Source: CAD feature listing. Evaluate the final solid. Frame: model axes, mm. Face numbers are marked on the shaded views. A direction names the side the tool comes from. Coordinates: 2 decimals unless noted, no trailing zeros. Loops run counter-clockwise (first coordinate to the right, second up) from the corner with the lowest first, then second, coordinate; pieces in that order, holes last. Notation, with made-up numbers: (59.5, -11.5) - (104.5, -11.5) arc R19 ccw to (104.5, 15.5) - close; hole circle Ø11 at (57.5, 19). An arc over 180 degrees is marked (long way). Use one line per item in the form item = value. Start each with the question number.
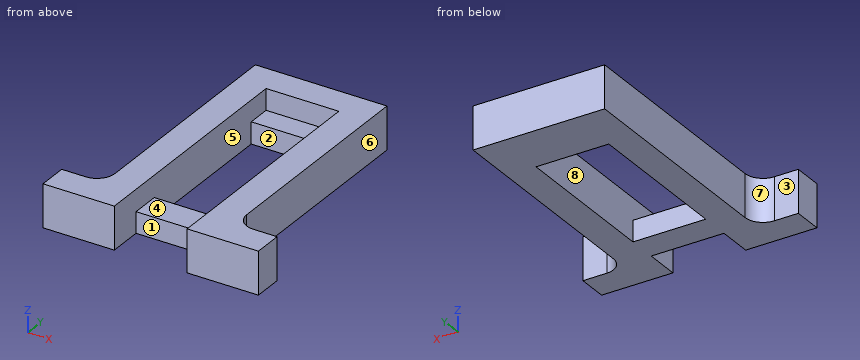
from build123d import *

# Parameters (mm, degrees)
F0_W     = 36
F0_H     = 44.84
F1_DEPTH = 7.13
F2_W     = 7
F2_H     = 39.92
F3_DEPTH = 7.13
F4_W     = 12.16
F4_H     = 36.01
F5_DEPTH = 7.13
F6_W     = 12.16
F6_H     = 3.91
F7_DEPTH = 3.53
F8_W     = 12.16
F8_H     = 4.8
F9_DEPTH = 3.5
F10_R    = 3


with BuildPart() as f1:
    # F0 (on Top) → F1 (new body)
    with BuildSketch(Plane.XY):
        with Locations((2.410514, 5.175292)):
            Rectangle(F0_W, F0_H)
    extrude(amount=F1_DEPTH)

    # F2 (on face) → F3 (cut)
    with BuildSketch(Plane.XY.offset(7.13)):
        with Locations((-12.089486, 7.635292)):
            Rectangle(F2_W, F2_H)
        with Locations((16.910514, 7.635292)):
            Rectangle(F2_W, F2_H)
    extrude(amount=-F3_DEPTH, mode=Mode.SUBTRACT)

    # F4 (on face) → F5 (cut)
    with BuildSketch(Plane.XY.offset(7.13)):
        with Locations((2.410514, 0.760292)):
            Rectangle(F4_W, F4_H)
    extrude(amount=-F5_DEPTH, mode=Mode.SUBTRACT)

    # F6 (on face) → F7 (cut)
    with BuildSketch(Plane.XY.offset(7.13)):
        with Locations((2.410514, 20.720292)):
            Rectangle(F6_W, F6_H)
    extrude(amount=-F7_DEPTH, mode=Mode.SUBTRACT)

    # F8 (on face) → F9 (join)
    with BuildSketch(Plane(origin=(0, 0, 0), x_dir=(1, 0, 0), z_dir=(0, 0, -1))):
        with Locations((2.410514, 9.134708)):
            Rectangle(F8_W, F8_H)
    extrude(amount=-F9_DEPTH)

    # F10
    f10_edges = [f1.edges().sort_by_distance(p)[0] for p in [
        (13.410514, -12.324708, 3.565),
        (-8.589486, -12.324708, 3.565),
    ]]
    fillet(f10_edges, radius=F10_R)


solid = f1.part
(1) Mould query, pull axis Y, two halves, no side actions, for the marked faces 6, 7 and 8. Classes: +Y half, -Y half, draft (parallel to the pull), parting line (faces both ways), or undercut.
(2) Cut plane D-D, the plane z = 6.25. Output: boundary loops of the cut face in (x, y).
(3) Contact query for flat-ended pins moving along their axis: pin 1 (1.2 mm diameter, centred on x = 4, y = 20.5, fed in from +Z); pin 2 (2 mm diameter, centred on y = -2, z = 1, fed in from +X); pin 3 (3 mm diameter, centred on x = 17.5, z = 4.5, fed in from +Y). Output: stop coordinate, or through.
(4) Material intervals for line 1 (X direction, y = 12, z = 4.25); line 2 (X direction, y = -15, z = 4.5); line 3 (Y direction, x = -1.5, z = 3.25), sorted ascending.
(5) Cut plane B-B, the plane x = 0. Output: boundary loops of the cut face in (y, z).
(6) Access query for the marked faces 1, 2, 3, 4 and 5. Directions: +Z, -Z, +X, -X, +Y, -Y. A direction counts if a zero-diameter tool reaches every point of the face in a straight line with its end or side. Return the directions, or none.
(7) Cut plane A-A, the plane y = -5.5. Output: boundary loops of the cut face in (x, z), plus the area to 3 significant figures.
(8) Cut plane C-C, the plane z = 0.75. Output: boundary loops of the cut face in (x, y), plus the area to 3 significant figures.
Recorded:
q1.face_6 = draft
q1.face_7 = +Y half
q1.face_8 = undercut
q2.outline = (-15.59, -17.24) - (-3.67, -17.24) - (-3.67, 22.68) - (8.49, 22.68) - (8.49, -17.24) - (20.41, -17.24) - (20.41, -12.32) - (16.41, -12.32) arc R3 cw to (13.41, -9.32) - (13.41, 27.6) - (-8.59, 27.6) - (-8.59, -9.32) arc R3 cw to (-11.59, -12.32) - (-15.59, -12.32) - close
q3.pin_1 = 3.6
q3.pin_2 = 13.41
q3.pin_3 = -12.3
q4.line_1 = -8.59 to -3.67, 8.49 to 13.41
q4.line_2 = -15.59 to -3.67, 8.49 to 20.41
q4.line_3 = -11.53 to -6.73, 18.77 to 27.6
q5.outline = (-11.53, 0) - (-6.73, 0) - (-6.73, 3.5) - (-11.53, 3.5) - close; (18.77, 0) - (27.6, 0) - (27.6, 7.13) - (22.68, 7.13) - (22.68, 3.6) - (18.77, 3.6) - close
q6.face_1 = +Z, -Z, -Y
q6.face_2 = +Z, -Z
q6.face_3 = +Z, -Z, -X, +Y
q6.face_4 = +Z, -Y
q6.face_5 = +Z
q7.outline = (-8.59, 0) - (-3.67, 0) - (-3.67, 7.13) - (-8.59, 7.13) - close; (8.49, 0) - (13.41, 0) - (13.41, 7.13) - (8.49, 7.13) - close
q7.area = 70.2 mm²
q8.outline = (-15.59, -17.24) - (-3.67, -17.24) - (-3.67, -11.53) - (8.49, -11.53) - (8.49, -17.24) - (20.41, -17.24) - (20.41, -12.32) - (16.41, -12.32) arc R3 cw to (13.41, -9.32) - (13.41, 27.6) - (-8.59, 27.6) - (-8.59, -9.32) arc R3 cw to (-11.59, -12.32) - (-15.59, -12.32) - close; hole (-3.67, -6.73) - (8.49, -6.73) - (8.49, 18.77) - (-3.67, 18.77) - close
q8.area = 680 mm²
